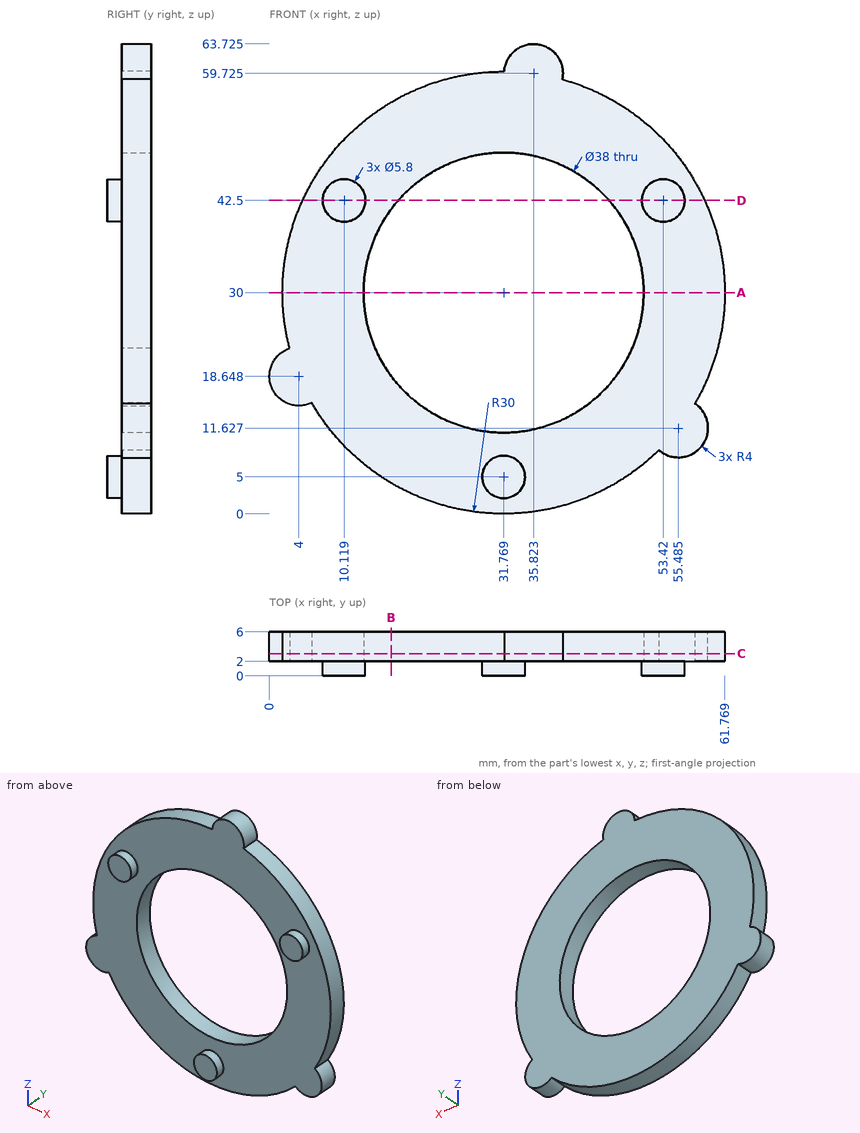
Answer from the drawing. Dimensions are ordinates in mm from the lowest x, y and z of the part. Coordinates: 2 decimals unless noted, no trailing zeros. Write each loop counter-clockwise with the first axis right and the second up, starting at its lowest first coordinate (ties: lowest second). Pieces come first, ordered by that corner, then holes. Notation, with made-up numbers: (63, -8) - (90, -8) arc R13 cw to (90, 4) - close; hole circle Ø7 at (-9, -30). An arc over 180 degrees is marked (long way). Return JSON: item names as keys, results as strings. Group by question number.
Q1. The part is cut by section A-A on z = 30. Write down the section's boundary in (x, y).
Q2. The part is cut by section D-D on z = 42.5. Write down the section's boundary in (x, y).
Q3. The part is cut by section B-B on x = 16.5. Write down the section's boundary in (y, z).
Q4. The part is cut by section C-C on y = 3.05. Write down the section's boundary in (x, z) (1 decimal).
Q5. Flat-ended cylindrical pins translate along their axes: pin 1 Ø1 at (x, y) = (45, 5) entering from +Z (1 decimal); pin 2 Ø1.5 at (x, y) = (16, 2.5) entering from +Z; pin 3 Ø1 at (y, z) = (2, 53.5) entering from +X; pin 4 Ø18.5 at (x, z) = (44, 43) entering from -Y. Find the tip coordinate at first contact, or state that the pin passes through.
Q6. Find the intervals of material crossed by line 1 along Z through (x, y) = (31, 3.45) (1 decimal); line 2 along X through (y, z) = (4.9, 30); line 3 along Z through (x, y) = (19, 2.45) (1 decimal), in increasing order. Write a range as [from, to].
Evaluation:
{
 "1": {"outline": "(1.77, 2) - (12.77, 2) - (12.77, 6) - (1.77, 6) - close; (50.77, 2) - (61.77, 2) - (61.77, 6) - (50.77, 6) - close"},
 "2": {"outline": "(4.5, 2) - (7.22, 2) - (7.22, 0) - (13.02, 0) - (13.02, 2) - (17.46, 2) - (17.46, 6) - (4.5, 6) - close; (46.08, 2) - (50.52, 2) - (50.52, 0) - (56.32, 0) - (56.32, 2) - (59.04, 2) - (59.04, 6) - (46.08, 6) - close"},
 "3": {"outline": "(2, 4.18) - (6, 4.18) - (6, 18.69) - (2, 18.69) - close; (2, 41.31) - (6, 41.31) - (6, 55.82) - (2, 55.82) - close"},
 "4": {"outline": "(2.7, 22.4) arc R4 ccw (long way) to (5.8, 15.1) arc R30 ccw to (52.8, 8.6) arc R4 ccw (long way) to (57.7, 14.9) arc R30 ccw to (39.7, 58.9) arc R4 ccw (long way) to (31.8, 60) arc R30 ccw to start; hole circle Ø38 at (31.8, 30)"},
 "5": {"pin 1": "stops at z = 57.2", "pin 2": "stops at z = 55.97", "pin 3": "stops at x = 51.03", "pin 4": "stops at y = 0"},
 "6": {"line 1": "z = [0, 11], [49, 60]", "line 2": "x = [1.77, 12.77], [50.77, 61.77]", "line 3": "z = [2.9, 15.9], [44.1, 57.1]"}
}
